Verification items for the finished model (mm, model axes). Face numbers are marked on the shaded views. Coordinates: 2 decimals unless noted, no trailing zeros. Loops run counter-clockwise (first coordinate to the right, second up) from the corner with the lowest first, then second, coordinate; pieces in that order, holes last. Notation, with made-up numbers: (70, 65.5) - (80, 65.5) arc R22 ccw to (80, 88.5) - close; hole circle Ø10 at (-5.5, 78.5). An arc over 180 degrees is marked (long way). Answer as CSV lines item,"result". Start each with the question number.
1. Release check for a two-part mould opening along Z. For the marked faces 1 and 2 record: pulls with the +Z half, pulls with the -Z half, needs draft (parallel to the pull), parting line crosses it, or undercut.
2. Material ranges on line 1 (X direction, y = -0.45, z = 0); line 2 (X direction, y = 2, z = 9.5); line 3 (Y direction, x = 2, z = 14), recorded low to high. Write a range as [from, to].
3. Gauge pin test, flat ends, axial feed: P1, Ø0.6, axis at y = 1, z = 0.5, coming from the +X side; P2, Ø6.5, axis at x = 0, z = 0, coming from the +Y side; P3, Ø1.7, axis at y = 0.5, z = -6.5, coming from the -X side. Record the tip position at first contact, or that the pin passes through.
4. Cross-section at B-B (z = 0). Enter the section's corners in (x, y).
5. Cross-section at D-D (x = 4.25). Enter the section's corners in (y, z), plus the area to 3 significant figures.
6. Cross-section at A-A (x = 0). Enter the section's corners in (y, z), plus the area to 3 significant figures.
7. Cross-section at C-C (z = 10). Enter the section's corners in (x, y), plus the area to 3 significant figures.
```python
from build123d import *
from build123d.topology import SkipClean

# Parameters (mm, degrees)
BOSS_EXTRUDE1_DEPTH = 2.1
BOSS_EXTRUDE2_START = -1.4
SKETCH2_R           = 2.5
BOSS_EXTRUDE2_DEPTH = 1.4
SKETCH4_W           = 13
SKETCH4_H           = 4.5
BOSS_EXTRUDE3_DEPTH = 42.2


with BuildPart() as part:
    # Sketch1 → Boss-Extrude1 (new body)
    with BuildSketch(Plane(origin=(0, 0, 0), x_dir=(1, 0, 0), z_dir=(0, 1, 0))):
        with BuildLine():
            Line((-5.75, 2.5), (-2.5, 5.75))
            Line((-2.5, 5.75), (-0.75, 5.75))
            Line((-0.75, 5.75), (-0.75, 7.964766161))
            ThreePointArc((-0.75, 7.964766161), (-7.280803408, 3.31510207), (-6.5, -4.663689527))
            Line((-6.5, -4.663689527), (-6.5, -15))
            Line((-6.5, -15), (6.5, -15))
            Line((6.5, -15), (6.5, -4.663689527))
            ThreePointArc((6.5, -4.663689527), (7.280803408, 3.31510207), (0.75, 7.964766161))
            Line((0.75, 7.964766161), (0.75, 5.75))
            Line((0.75, 5.75), (2.5, 5.75))
            Line((2.5, 5.75), (5.75, 2.5))
            Line((5.75, 2.5), (5.75, -6.75))
            Line((5.75, -6.75), (-5.75, -6.75))
            Line((-5.75, -6.75), (-5.75, 2.5))
        make_face()
    extrude(amount=BOSS_EXTRUDE1_DEPTH)

    # Sketch2 → Boss-Extrude2 (add)
    with SkipClean():  # the faces are left unmerged after this step: merging them gives an invalid solid
        with BuildSketch(Plane(origin=(0, 0, 0), x_dir=(1, 0, 0), z_dir=(0, 1, 0)).offset(BOSS_EXTRUDE2_START)):
            with BuildLine():
                Line((6.5, -4.663689527), (6.5, -15))
                Line((6.5, -15), (-6.5, -15))
                Line((-6.5, -15), (-6.5, -4.663689527))
                ThreePointArc((-6.5, -4.663689527), (0, 8), (6.5, -4.663689527))
            make_face()
            with Locations(Location((0, 0, 0), (0, 0, 270))):
                Circle(SKETCH2_R, mode=Mode.SUBTRACT)
            with BuildLine():
                Line((-5, -5.5), (-5, -6.75))
                Line((-5, -6.75), (-3.5, -6.75))
                Line((-3.5, -6.75), (-3.5, -5.5))
                ThreePointArc((-3.5, -5.5), (-4.25, -4.75), (-5, -5.5))
            make_face(mode=Mode.SUBTRACT)
            with BuildLine():
                Line((3.5, -5.5), (3.5, -6.75))
                Line((3.5, -6.75), (5, -6.75))
                Line((5, -6.75), (5, -5.5))
                ThreePointArc((5, -5.5), (4.25, -4.75), (3.5, -5.5))
            make_face(mode=Mode.SUBTRACT)
        extrude(amount=BOSS_EXTRUDE2_DEPTH)

    # Sketch4 → Boss-Extrude3 (add)
    with SkipClean():  # the faces are left unmerged after this step: merging them gives an invalid solid
        with BuildSketch(Plane.XY.offset(15)):
            with Locations((0, 0.85)):
                Rectangle(SKETCH4_W, SKETCH4_H)
        extrude(amount=BOSS_EXTRUDE3_DEPTH)


solid = part.part
```
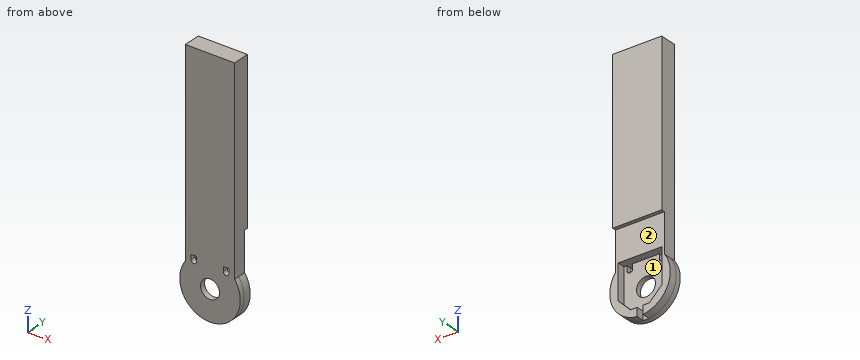
Values follow:
1,face 1,"undercut"
1,face 2,"needs draft"
2,line 1,"x = [-8, -2.5], [2.5, 8]"
2,line 2,"x = [-6.5, 6.5]"
2,line 3,"y = [-1.4, 2.1]"
3,P1,"stops at x = 8"
3,P2,"stops at y = 0"
3,P3,"stops at x = -5.66"
4,outline,"(-8, -1.4) - (-2.5, -1.4) - (-2.5, 0) - (-5.75, 0) - (-5.75, 2.1) - (-8, 2.1) - close; (2.5, -1.4) - (8, -1.4) - (8, 2.1) - (5.75, 2.1) - (5.75, 0) - (2.5, 0) - close"
5,outline,"(-1.4, -6.78) - (2.1, -6.78) - (2.1, -4) - (0, -4) - (0, 4.75) - (-1.4, 4.75) - close; (-1.4, 6.75) - (2.1, 6.75) - (2.1, 15) - (3.1, 15) - (3.1, 57.2) - (-1.4, 57.2) - close"
5,area,"241 mm²"
6,outline,"(-1.4, -8) - (0, -8) - (0, -2.5) - (-1.4, -2.5) - close; (-1.4, 2.5) - (0, 2.5) - (0, 6.75) - (2.1, 6.75) - (2.1, 15) - (3.1, 15) - (3.1, 57.2) - (-1.4, 57.2) - close"
6,area,"232 mm²"
7,outline,"(-6.5, -1.4) - (6.5, -1.4) - (6.5, 2.1) - (-6.5, 2.1) - close"
7,area,"45.5 mm²"
